Source: three-view drawing plus pictorial views. Frame: mm from the lowest corner of the part. Give positions to 0.01 mm unless a question says otherwise; leave off trailing zeros. Order: outer loops, then holes, each group sorted by start corner. A loop starts at its lowest first (then second) coordinate and runs counter-clockwise, first axis right, second up. Notation, with made-up numbers: (38, 86.25) - (68, 86.25) arc R21 ccw to (68, 95.25) - close; hole circle Ø1 at (-26.5, 10.25). An arc over 180 degrees is marked (long way). Answer in a Markdown table with one row per item. Add a question column.
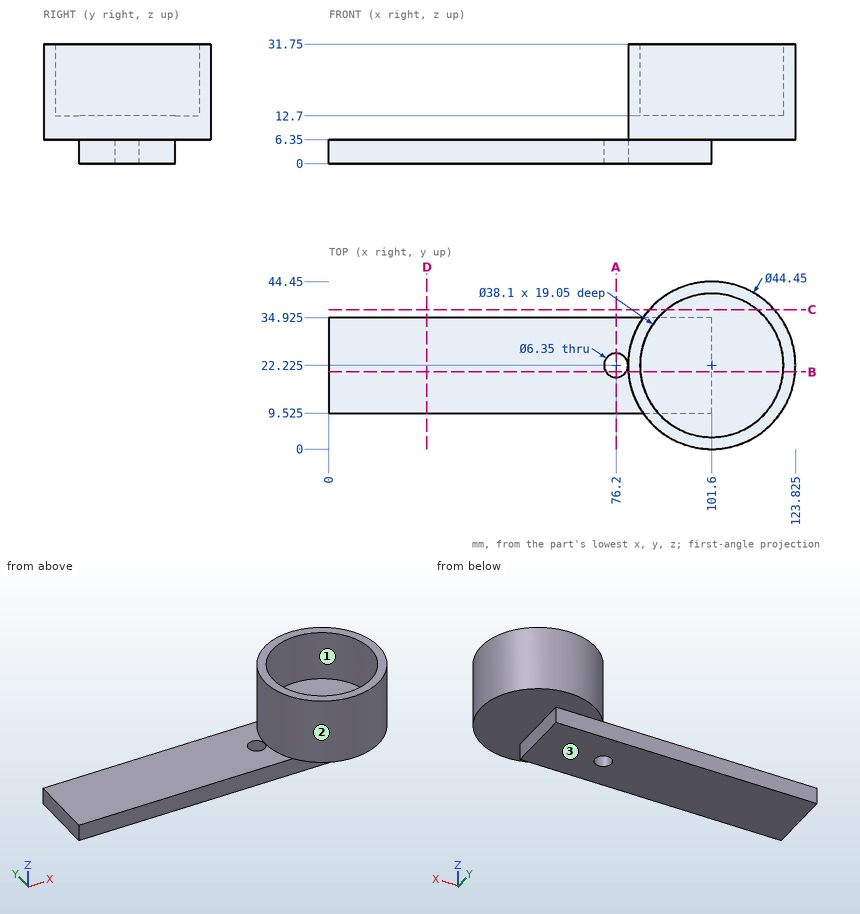
Q1. Line query: probe 1 along Y at (x, z) = (76, 3) (3 decimals); probe 2 along Z at (x, y) = (103.5, 12); probe 3 along Y at (x, z) = (36, 3) (3 decimals). Output: solid intervals per line, ascending.
Q2. Pull-direction query (Y, two-part tool) for the marked faces 1, 2 and 3; classes: +Y half, -Y half, draft (parallel to the pull), parting line (faces both ways), or undercut.
Q3. Section C-C, the plane y = 37. Return loops of the section in (x, z).
Q4. Section D-D, the plane x = 26. Return loops of the section in (y, z) (3 decimals).
Q5. Contact query for flat-ended pins moving along their axis: P1, Ø2, axis at x = 58, y = 28, coming from the +Z side; P2, Ø3, axis at x = 69.5, z = 2, coming from the -Y side (3 decimals); P3, Ø1.5, axis at y = 33.5, z = 3.5, coming from the +X side. Output: stop coordinate, or through.
Q6. Section A-A, the plane x = 76.2. Return loops of the section in (y, z) (3 decimals).
Q7. Section B-B, the plane y = 20.5. Return loops of the section in (x, z).
Computed:
| question | item | result |
|---|---|---|
| 1 | probe 1 | y = 9.525 to 19.056, 25.394 to 34.925 |
| 1 | probe 2 | z = 6.35 to 12.7 |
| 1 | probe 3 | y = 9.525 to 34.925 |
| 2 | face 1 | undercut |
| 2 | face 2 | parting line |
| 2 | face 3 | draft |
| 3 | outline | (85, 6.35) - (118.2, 6.35) - (118.2, 31.75) - (113.63, 31.75) - (113.63, 12.7) - (89.57, 12.7) - (89.57, 31.75) - (85, 31.75) - close |
| 4 | outline | (9.525, 0) - (34.925, 0) - (34.925, 6.35) - (9.525, 6.35) - close |
| 5 | P1 | stops at z = 6.35 |
| 5 | P2 | stops at y = 9.525 |
| 5 | P3 | stops at x = 101.6 |
| 6 | outline | (9.525, 0) - (19.05, 0) - (19.05, 6.35) - (9.525, 6.35) - close; (25.4, 0) - (34.925, 0) - (34.925, 6.35) - (25.4, 6.35) - close |
| 7 | outline | (0, 0) - (73.53, 0) - (73.53, 6.35) - (0, 6.35) - close; (78.87, 0) - (101.6, 0) - (101.6, 6.35) - (123.76, 6.35) - (123.76, 31.75) - (120.57, 31.75) - (120.57, 12.7) - (82.63, 12.7) - (82.63, 31.75) - (79.44, 31.75) - (79.44, 6.35) - (78.87, 6.35) - close |
